Can you work these out from the model? Positions are in its coordinate system, mm. A direction names the side the tool comes from. Round coordinates to 2 decimals unless told otherwise and drop trailing zeros. Loops run counter-clockwise (first coordinate to the right, second up) from the corner with the lowest first, then second, coordinate; pieces in that order, holes last. Notation, with made-up numbers: (47.5, -39) -> (104.5, -39) arc R27 cw to (104.5, -5) -> close; hole circle Ø4 at (86.5, 52). An arc over 180 degrees is marked (long way). Use a Markdown table: item, result.
from build123d import *

# Parameters (mm, degrees)
F0_R      = 26
F1_DEPTH  = 7.6
F3_R      = 28.5
F4_DEPTH  = 17.7
F6_R      = 4
F7_DEPTH  = 45.4
F9_R      = 2.4
F10_DEPTH = 29.8


with BuildPart() as f1:
    # F0 (on Top) → F1 (new body)
    with BuildSketch(Plane.XY):
        Circle(F0_R)
    extrude(amount=-F1_DEPTH)

    # F3 (on offset) → F4 (join, through all)
    with BuildSketch(Plane.XY.offset(17.7)):
        Circle(F3_R)
    extrude(amount=-F4_DEPTH)

    # F6 (on Front) → F7 (join, through all)
    with BuildSketch(Plane.XZ):
        Circle(F6_R)
    extrude(amount=F7_DEPTH)

    # F9 (on face) → F10 (join, through all)
    with BuildSketch(Plane.XZ.offset(45.4)):
        Circle(F9_R)
    extrude(amount=F10_DEPTH)


solid = f1.part
1. Which directions (+Z, -Z, +X, -X, +Y, -Y) give clear straight access to the entire face, cutting with the end or side of a thin tool? Please do faces 1 (the flat face through (0, 0, -7.6)), 2 (the cylindrical face through (1.29, -60.091, 2.024)), 3 (the flat face through (23.1, -12.3, 0)).
Answer sheet:
| item | result |
|---|---|
| face 1 | -Z, +X, -X, +Y, -Y |
| face 2 | -Y |
| face 3 | -Z |
2. I want a section at A-A (y = 0). Please give me the cut outline in (x, z), plus the area to 3 significant figures.
Answer sheet:
| item | result |
|---|---|
| outline | (-28.5, 0) -> (-26, 0) -> (-26, -7.6) -> (26, -7.6) -> (26, 0) -> (28.5, 0) -> (28.5, 17.7) -> (-28.5, 17.7) -> close |
| area | 1,400 mm² |
3. I want a section at B-B (x = 0). Please give me the cut outline in (y, z), plus the area to 3 significant figures.
Answer sheet:
| item | result |
|---|---|
| outline | (-75.2, -2.4) -> (-45.4, -2.4) -> (-45.4, -4) -> (-26, -4) -> (-26, -7.6) -> (26, -7.6) -> (26, 0) -> (28.5, 0) -> (28.5, 17.7) -> (-28.5, 17.7) -> (-28.5, 4) -> (-45.4, 4) -> (-45.4, 2.4) -> (-75.2, 2.4) -> close |
| area | 1,690 mm² |
4. I want a section at D-D (x = 19.5). Please give me the cut outline in (y, z), plus the area to 3 significant figures.
Answer sheet:
| item | result |
|---|---|
| outline | (-20.78, 0) -> (-17.2, 0) -> (-17.2, -7.6) -> (17.2, -7.6) -> (17.2, 0) -> (20.78, 0) -> (20.78, 17.7) -> (-20.78, 17.7) -> close |
| area | 997 mm² |
5. Will these pins go through, and if not, where does the flat tip stop? pin 1 Ø12 at (x, z) = (-2, -3.5) entering from +Y; pin 2 Ø6 at (y, z) = (3, 5.5) entering from +X; pin 3 Ø1.5 at (x, z) = (-10, 12.5) entering from +Y; pin 4 Ø6 at (y, z) = (13, 1) entering from +X.
Answer sheet:
| item | result |
|---|---|
| pin 1 | stops at y = 28.5 |
| pin 2 | stops at x = 28.5 |
| pin 3 | stops at y = 26.96 |
| pin 4 | stops at x = 26.69 |
6. I need wall thicknesses on line 1 (X direction, y = -65.5, z = -0.25); line 2 (Y direction, x = -0.5, z = 4); line 3 (X direction, y = 9.5, z = 8.25). Which ranges of each line are inside material? Lowest first, please.
Answer sheet:
| item | result |
|---|---|
| line 1 | x = -2.39 to 2.39 |
| line 2 | y = -28.5 to 28.5 |
| line 3 | x = -26.87 to 26.87 |
7. I want a section at C-C (z = 11). Please give me the cut outline in (x, y), plus the area to 3 significant figures.
Answer sheet:
| item | result |
|---|---|
| outline | circle Ø57 at (0, 0) |
| area | 2,550 mm² |
